from build123d import *

# Parameters (mm, degrees)
F0_R     = 1.5
F0_R_2   = 4
F0_R_3   = 6
F1_DEPTH = 28


# Not quite as in the source:
# - ends of sketch curves that miss each other by under 0.0002 mm in the source are joined


with BuildPart() as f1:
    # F0 (on Top) → F1 (new body)
    with BuildSketch(Plane.XY):
        with BuildLine():
            ThreePointArc((-46.3352200183, -18.0903971195), (-28.5000011764, -13.2245283483), (-10.6647820085, -18.0903959247))
            ThreePointArc((-10.6647820085, -18.0903959247), (21, 0), (-10.6647820085, 18.0903959247))
            ThreePointArc((-10.6647820085, 18.0903959247), (-28.5000011764, 13.2245283483), (-46.3352200183, 18.0903971195))
            ThreePointArc((-46.3352200183, 18.0903971195), (-57.0000007926, 21), (-67.6647813473, 18.0903963145))
            ThreePointArc((-67.6647813473, 18.0903963145), (-85.5000011764, 13.2245283483), (-103.3352200183, 18.0903971195))
            ThreePointArc((-103.3352200183, 18.0903971195), (-112.7285298393, 20.9614733173), (-122.4, 19.2468179188))
            Line((-122.4, 19.2468179188), (-156, 4.582575695))
            ThreePointArc((-156, 4.582575695), (-159, 0), (-156, -4.582575695))
            Line((-156, -4.582575695), (-122.4, -19.2468179188))
            ThreePointArc((-122.4, -19.2468179188), (-112.7285306305, -20.9614733653), (-103.3352200183, -18.0903971195))
            ThreePointArc((-103.3352200183, -18.0903971195), (-85.5000011764, -13.2245283483), (-67.6647820085, -18.0903959247))
            ThreePointArc((-67.6647820085, -18.0903959247), (-57.0000011764, -21), (-46.3352200183, -18.0903971195))
        make_face()
        with Locations((-154, 0)):
            Circle(F0_R, mode=Mode.SUBTRACT)
        with Locations((-114, 0)):
            Circle(F0_R_2, mode=Mode.SUBTRACT)
        with Locations((-57, 0)):
            Circle(F0_R_3, mode=Mode.SUBTRACT)
        Circle(F0_R_2, mode=Mode.SUBTRACT)
    extrude(amount=F1_DEPTH)


solid = f1.part
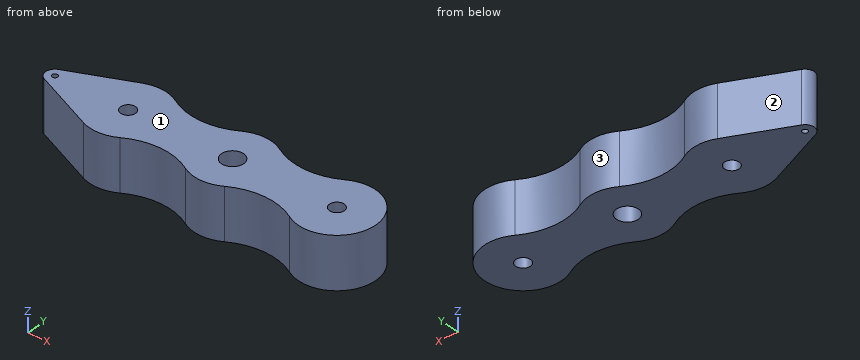
Verification items for the finished model (mm, model axes). Face numbers are marked on the shaded views. Give positions to 0.01 mm unless a question says otherwise; leave off trailing zeros. Write each loop counter-clockwise with the first axis right and the second up, starting at its lowest first coordinate (ties: lowest second). Pieces come first, ordered by that corner, then holes.
(1) Material ranges on line 1 (Y direction, x = -57, z = 21.5); line 2 (Y direction, x = -114, z = 10); line 3 (X direction, y = 3, z = 17), recorded low to high.
(2) Cross-section at C-C (z = 17.25). Enter the section's corners in (x, y).
(3) Cross-section at B-B (y = 0). Enter the section's corners in (x, z).
(4) Mould release check, pull along X, two halves, no side actions. Record for the marked faces 1, 2 and 3: +X half, -X half, draft (parallel to the pull), parting line (faces both ways), or undercut.
(5) Gauge pin test, flat ends, axial feed: pin 1 (1.5 mm diameter, centred on y = -10.5, z = 6, fed in from -X); pin 2 (1.8 mm diameter, centred on x = -154, y = 0, fed in from -Z); pin 3 (1.5 mm diameter, centred on x = -68, z = 7.5, fed in from -Y); pin 4 (12 mm diameter, centred on y = 6.5, z = 15.5, fed in from +X). Record the tip position at first contact, or that the pin passes through.
(6) Cross-section at D-D (x = -114). Enter the section's corners in (y, z), plus the area to 3 significant figures.
(7) Cross-section at A-A (x = -57). Enter the section's corners in (y, z).
Worked out:
1. line 1: y = -21 to -6, 6 to 21
1. line 2: y = -21 to -4, 4 to 21
1. line 3: x = -158 to -116.65, -111.35 to -62.2, -51.8 to -2.65, 2.65 to 20.78
2. outline: (-156, -4.58) - (-122.4, -19.25) arc R21 ccw to (-103.34, -18.09) arc R35.12 cw to (-67.66, -18.09) arc R21 ccw to (-46.34, -18.09) arc R35.12 cw to (-10.66, -18.09) arc R21 ccw (long way) to (-10.66, 18.09) arc R35.12 cw to (-46.34, 18.09) arc R21 ccw to (-67.66, 18.09) arc R35.12 cw to (-103.34, 18.09) arc R21 ccw to (-122.4, 19.25) - (-156, 4.58) arc R5 ccw to start; hole circle Ø3 at (-154, 0); hole circle Ø8 at (-114, 0); hole circle Ø12 at (-57, 0); hole circle Ø8 at (0, 0)
3. outline: (-159, 0) - (-155.5, 0) - (-155.5, 28) - (-159, 28) - close; (-152.5, 0) - (-118, 0) - (-118, 28) - (-152.5, 28) - close; (-110, 0) - (-63, 0) - (-63, 28) - (-110, 28) - close; (-51, 0) - (-4, 0) - (-4, 28) - (-51, 28) - close; (4, 0) - (21, 0) - (21, 28) - (4, 28) - close
4. face 1: draft
4. face 2: -X half
4. face 3: undercut
5. pin 1: stops at x = -144.16
5. pin 2: passes through
5. pin 3: stops at y = -18.33
5. pin 4: stops at x = 20.99
6. outline: (-21, 0) - (-4, 0) - (-4, 28) - (-21, 28) - close; (4, 0) - (21, 0) - (21, 28) - (4, 28) - close
6. area: 952 mm2
7. outline: (-21, 0) - (-6, 0) - (-6, 28) - (-21, 28) - close; (6, 0) - (21, 0) - (21, 28) - (6, 28) - close
